Autodesk Inventor part; units mm, degrees
ref_plane "YZ Plane" through (0, 0, 0) normal (1, 0, 0) x (0, 1, 0)
ref_plane "XZ Plane" through (0, 0, 0) normal (0, 1, 0) x (-1, 0, 0)
ref_plane "XY Plane" through (0, 0, 0) normal (0, 0, 1) x (1, 0, 0)
sketch "Szkic1" plane through (0, 0, 0) normal (0, 1, 0) x (-1, 0, 0)
  line L0 (0, 0) -> (88, 0)
  line L1 (88, 0) -> (88, 64.5)
  line L2 (88, 64.5) -> (0, 64.5)
  line L3 (0, 64.5) -> (0, 0)
  line L4 (88, 64.5) -> (86.5, 64.5) construction
  line L5 (86.5, 64.5) -> (86.5, 63) construction
  line L6 (86.5, 63) -> (88, 63) construction
  line L7 (88, 63) -> (88, 64.5) construction
  line L8 (0, 0) -> (1.5, 0) construction
  line L9 (1.5, 0) -> (1.5, 1.5) construction
  line L10 (1.5, 1.5) -> (0, 1.5) construction
  line L11 (0, 1.5) -> (0, 0) construction
  line L12 (86.5, 63) -> (1.5, 63)
  line L13 (1.5, 63) -> (1.5, 1.5)
  line L14 (1.5, 1.5) -> (86.5, 1.5)
  line L15 (86.5, 1.5) -> (86.5, 63)
  dimension "d0" = 88
  dimension "d1" = 64.5
  dimension "d2" = 1.5
  dimension "d3" = 1.5
  dimension "d4" = 1.5
  dimension "d5" = 1.5
extrude "Wyciągnięcie proste1" add sketch "Szkic1" against normal blind 2
sketch "Szkic2" plane through (0, 0, 0) normal (0, 1, 0) x (1, 0, 0)
  line L0 (0, -64.5) -> (-88, -64.5) construction
  line L1 (0, -64.5) -> (1.5, -64.5) construction
  line L2 (1.5, -64.5) -> (1.5, -69) construction
  line L3 (1.5, -69) -> (0, -69) construction
  line L4 (0, -69) -> (0, -64.5) construction
  line L5 (-88, 0) -> (0, 0) construction
  line L6 (-88, 0) -> (-89.5, 0) construction
  line L7 (-89.5, 0) -> (-89.5, 4.5) construction
  line L8 (-89.5, 4.5) -> (-88, 4.5) construction
  line L9 (-88, 4.5) -> (-88, 0) construction
  line L10 (1.5, -69) -> (-89.5, -69)
  line L11 (-89.5, -69) -> (-89.5, 4.5)
  line L12 (-89.5, 4.5) -> (1.5, 4.5)
  line L13 (1.5, 4.5) -> (1.5, -69)
  line L14 (-86.5, -1.5) -> (-86.5, -63)
  line L15 (-1.5, -63) -> (-86.5, -63)
  line L16 (-86.5, -63) -> (-86.5, -1.5)
  line L17 (-86.5, -1.5) -> (-1.5, -1.5)
  line L18 (-1.5, -1.5) -> (-1.5, -63)
  dimension "d8" = 1.5
  dimension "d9" = 4.5
  dimension "d10" = 1.5
  dimension "d11" = 4.5
extrude "Wyciągnięcie proste2" add sketch "Szkic2" along normal blind 1
sketch "Szkic3" plane through (0, 1, 0) normal (0, 1, 0) x (1, 0, 0)
  line L0 (-89.5, -69) -> (1.5, -69) construction
  line L1 (1.5, -69) -> (0, -69) construction
  line L2 (0, -69) -> (0, -67.5) construction
  line L3 (0, -67.5) -> (1.5, -67.5) construction
  line L4 (1.5, -67.5) -> (1.5, -69) construction
  line L5 (-89.5, 4.5) -> (-89.5, -69) construction
  line L6 (-89.5, 4.5) -> (-88, 4.5) construction
  line L7 (-88, 4.5) -> (-88, 3) construction
  line L8 (-88, 3) -> (-89.5, 3) construction
  line L9 (-89.5, 3) -> (-89.5, 4.5) construction
  line L10 (0, -67.5) -> (-88, -67.5)
  line L11 (-88, -67.5) -> (-88, 3)
  line L12 (-88, 3) -> (0, 3)
  line L13 (0, 3) -> (0, -67.5)
  line L14 (1.5, 4.5) -> (-89.5, 4.5)
  line L15 (1.5, -69) -> (-89.5, -69)
  line L16 (-89.5, -69) -> (-89.5, 4.5)
  line L17 (-89.5, 4.5) -> (1.5, 4.5)
  line L18 (1.5, 4.5) -> (1.5, -69)
  point P0 (0, 0)
  dimension "d14" = 1.5
  dimension "d15" = 1.5
  dimension "d16" = 1.5
  dimension "d17" = 1.5
extrude "Wyciągnięcie proste3" add sketch "Szkic3" along normal blind 27
sketch "Szkic4" plane through (0, 1, -3) normal (-1, 0, 0) x (0, 0, 1)
  line L0 (72, -1) -> (67.5, -1)
  line L1 (67.5, -1) -> (3, -1)
  line L2 (3, -1) -> (-1.5, -1)
  line L3 (-1.5, -1) -> (-1.5, 27)
  line L4 (-1.5, 27) -> (0, 27)
  line L5 (0, 27) -> (70.5, 27)
  line L6 (70.5, 27) -> (72, 27)
  line L7 (72, 27) -> (72, -1)
  line L8 (67.5, -1) -> (67.5, -3)
  line L9 (67.5, -3) -> (3, -3)
  line L10 (3, -3) -> (3, -1)
  line L11 (0, 27) -> (0, 0)
  line L12 (0, 0) -> (70.5, 0)
  line L13 (70.5, 0) -> (70.5, 27)
  line L14 (72, -1) -> (67.5, -1)
  line L15 (67.5, -1) -> (3, -1)
  line L16 (3, -1) -> (-1.5, -1)
  line L17 (-1.5, -1) -> (-1.5, 27)
  line L18 (-1.5, 27) -> (0, 27)
  line L19 (0, 27) -> (70.5, 27)
  line L20 (70.5, 27) -> (72, 27)
  line L21 (72, 27) -> (72, -1)
  line L22 (67.5, -1) -> (67.5, -3)
  line L23 (67.5, -3) -> (3, -3)
  line L24 (3, -3) -> (3, -1)
  line L25 (0, 27) -> (0, 0)
  line L26 (0, 0) -> (70.5, 0)
  line L27 (70.5, 0) -> (70.5, 27)
  line L28 (0, 0) -> (8.65, 0) construction
  line L29 (70.5, 0) -> (0, 0) construction
  line L30 (8.65, 0) -> (24.95, 0) construction
  line L31 (8.65, 0) -> (24.95, 0)
  line L32 (24.95, 0) -> (24.95, 27)
  line L33 (24.95, 27) -> (8.65, 27)
  line L34 (8.65, 27) -> (8.65, 0)
  dimension "d20" = 8.65
  dimension "d21" = 16.3
extrude "Wyciągnięcie proste4" cut sketch "Szkic4" against normal blind 1.5 contours L32 L12 L34 L5
sketch "Szkic5" plane through (0, 1, 0) normal (0, 1, 0) x (1, 0, 0)
  line L0 (-88, 3) -> (-88, -67.5) construction
  line L1 (-88, 3) -> (-88, -30.9) construction
  line L2 (-88, -30.9) -> (-86.5, -30.9)
  line L3 (-86.5, -30.9) -> (-86.5, -33.9)
  line L4 (-86.5, -33.9) -> (-88, -33.9)
  line L5 (-88, -33.9) -> (-88, -30.9)
  point P0 (0, 0)
  dimension "d24" = 33.9
  dimension "d25" = 1.5
  dimension "d26" = 3
extrude "Wyciągnięcie proste5" add sketch "Szkic5" along normal blind 27
sketch "Szkic6" plane through (0, 1, 0) normal (0, 1, 0) x (1, 0, 0)
  line L0 (-1.5, -1.5) -> (-1.5, -63) construction
  line L1 (-1.5, -63) -> (-1.5, -26) construction
  line L2 (-1.5, -63) -> (-16.5, -63) construction
  line L3 (-1.5, -63) -> (-86.5, -63) construction
  line L4 (-1.5, -26) -> (-1.5, -63)
  line L5 (-16.5, -63) -> (-1.5, -63)
  line L6 (-16.5, -63) -> (-16.5, -67.5)
  line L7 (0, -67.5) -> (-88, -67.5)
  line L8 (-16.5, -67.5) -> (0, -67.5)
  line L9 (0, -67.5) -> (0, -26)
  line L10 (0, -21.95) -> (0, -67.5)
  line L11 (-1.5, -26) -> (0, -26)
  point P0 (0, 0)
  dimension "d29" = 37
  dimension "d30" = 15
extrude "Wyciągnięcie proste6" add sketch "Szkic6" along normal blind 25
properties part number "gora"
Read the model definition and answer for the solid it produces. Units are mm, in the model's axes. A direction names the side the tool comes from. Coordinates: 2 decimals unless noted, no trailing zeros. Loops run counter-clockwise (first coordinate to the right, second up) from the corner with the lowest first, then second, coordinate; pieces in that order, holes last.
Q1. The mould has two halves that part along X. Classify faces 1 (the face through (-45, -1, 64.5)), 2 (the face through (-89.5, 14, 33)), 3 (the face through (-22.2, 0.5, 63)): +X half, -X half, draft (parallel to the pull), parting line (faces both ways), or undercut.
Q2. Which of the six approach directions +Z, -Z, +X, -X, +Y, -Y give full straight-line access (tool end or side, diameter ignored) to faces 4 (the face through (-43, -1, 0)), 5 (the face through (-45, 14, -3)), 6 (the face through (0, -1, 33)), 7 (the face through (-43, 0, 1.5)), 8 (the face through (-88, -1, 32))?
Q3. The part is cut by section A-A on z = 16.5. Write down the section's boundary in (x, y).
Q4. Each of these flat-tipped pins is pushed along its axis until it touches: pin 1 Ø0.6 at (y, z) = (-1, 33) entering from +X; pin 2 Ø0.6 at (x, y) = (-65, -1) entering from +Z. Where does it stop, or does it pass through?
Q5. The part is cut by section D-D on z = 54. Write down the section's boundary in (x, y), and give its area (4 significant figures).
Q6. The part is cut by section B-B on x = -29.5. Write down the section's boundary in (y, z), and give its area (3 significant figures).
Q7. The part is cut by section C-C on y = 23.75. Write down the section's boundary in (x, z).
Q8. Consider probe 1 along X at (y, z) = (18, 28); probe 2 along Z at (x, y) = (-45, 17.75); probe 3 along X at (y, z) = (26.5, -1). Determine where each line is inside the solid, lowest interval first.
Results below:
1. face 1: draft
1. face 2: -X half
1. face 3: undercut
2. face 4: -Z, +X, -X, -Y
2. face 5: +Y
2. face 6: +Z, -Z, +X, -Y
2. face 7: +Y, -Y
2. face 8: +Z, -Z, -X, -Y
3. outline: (-89.5, 0) - (-88, 0) - (-88, -2) - (-86.5, -2) - (-86.5, 1) - (-88, 1) - (-88, 28) - (-89.5, 28) - close; (-1.5, -2) - (0, -2) - (0, 0) - (1.5, 0) - (1.5, 1) - (-1.5, 1) - close
4. pin 1: stops at x = 0
4. pin 2: stops at z = 64.5
5. outline: (-89.5, 0) - (-88, 0) - (-88, -2) - (-86.5, -2) - (-86.5, 1) - (-88, 1) - (-88, 28) - (-89.5, 28) - close; (-1.5, -2) - (0, -2) - (0, 0) - (1.5, 0) - (1.5, 28) - (0, 28) - (0, 26) - (-1.5, 26) - close
5. area: 130.5 mm2
6. outline: (-2, 0) - (0, 0) - (0, -4.5) - (28, -4.5) - (28, -3) - (1, -3) - (1, 1.5) - (-2, 1.5) - close; (-2, 63) - (1, 63) - (1, 67.5) - (28, 67.5) - (28, 69) - (0, 69) - (0, 64.5) - (-2, 64.5) - close
6. area: 99.0 mm2
7. outline: (-89.5, -4.5) - (1.5, -4.5) - (1.5, 5.65) - (0, 5.65) - (0, -3) - (-88, -3) - (-88, 30.9) - (-86.5, 30.9) - (-86.5, 33.9) - (-88, 33.9) - (-88, 67.5) - (-16.5, 67.5) - (-16.5, 63) - (-1.5, 63) - (-1.5, 26) - (0, 26) - (0, 21.95) - (1.5, 21.95) - (1.5, 69) - (-89.5, 69) - close
8. probe 1: x = -89.5 to -88, -1.5 to 1.5
8. probe 2: z = -4.5 to -3, 67.5 to 69
8. probe 3: x = -89.5 to -88, 0 to 1.5
